Design review of the part built by this model. Coordinates are the model's own, in mm. Give positions to 0.01 mm unless a question says otherwise; leave off trailing zeros. Order: outer loops, then holes, each group sorted by start corner. A loop starts at its lowest first (then second) coordinate and runs counter-clockwise, first axis right, second up. Notation, with made-up numbers: M -26.5,82 L -18.5,82 A12 cw -18.5,86 Z; hole C 35.5,-8 d2. An arc over 180 degrees is marked long. Put each result on its own line as item: value. Start each with the question number.
Autodesk Inventor part; units mm, degrees
ref_plane "YZ Plane" through (0, 0, 0) normal (1, 0, 0) x (0, 1, 0)
ref_plane "XZ Plane" through (0, 0, 0) normal (0, 1, 0) x (-1, 0, 0)
ref_plane "XY Plane" through (0, 0, 0) normal (0, 0, 1) x (1, 0, 0)
sketch "Sketch1" plane through (0, 0, 0) normal (0, 0, 1) x (1, 0, 0)
  circle A0 centre (0, 0) radius 3.4
  line L0 (1.1333, -3.7357) -> (-1.1333, -3.7357)
  line L1 (-1.5333, -3.3357) -> (-1.5333, 3.3357)
  line L2 (-1.1333, 3.7357) -> (1.1333, 3.7357)
  line L3 (1.5333, 3.3357) -> (1.5333, -3.3357)
  line L4 (1.5333, -3.7357) -> (-1.5333, 3.7357) construction
  line L5 (-1.5333, -3.7357) -> (1.5333, 3.7357) construction
  arc A1 (-1.1333, 3.7357) -> (-1.5333, 3.3357) centre (-1.1333, 3.3357) ccw
  arc A2 (1.5333, 3.3357) -> (1.1333, 3.7357) centre (1.1333, 3.3357) ccw
  arc A3 (1.1333, -3.7357) -> (1.5333, -3.3357) centre (1.1333, -3.3357) ccw
  arc A4 (-1.5333, -3.3357) -> (-1.1333, -3.7357) centre (-1.1333, -3.3357) ccw
  point P0 (-1.5333, 3.0346)
  point P1 (-1.5333, -3.0346)
  point P2 (1.5333, -3.0346)
  point P3 (1.5333, 3.0346)
  point P4 (-0.9416, 2.2076)
  point P5 (-0.9416, -2.2076)
  point P6 (0.9416, -2.2076)
  point P7 (0.9416, 2.2076)
  dimension "d0" = 6.8
  dimension "d1" = 3.0667
  dimension "d2" = 7.4714
  dimension "d3" = 0.4
extrude "Extrusion1" add sketch "Sketch1" along normal blind 30
equation "\"d0\" = D_axel - d_toleransAxel"
equation "\"d3\" = r_filletAxel"
equation "\"d4\" = h_axel"
equation "\"D_axel\" = D_axel_1"
equation "\"d_axelRing\" = d_axelRing_1"
equation "\"r_filletAxel\" = r_filletAxel_1"
equation "\"d_toleransAxel\" = 0.2"
equation "\"h_axel\" = 30"
properties part number "Axel_parametriserad_03"
1. Consider section A-A on z = 25. Give the boundary of the cut face in (x, y).
2. Consider section B-B on y = 2.5. Give the boundary of the cut face in (x, z), then the cut area to 3 significant figures.
3. To check wall thickness, follow probe 1 along X at (y, z) = (0.25, 22.5); probe 2 along Y at (x, z) = (1.25, 4); probe 3 along Y at (x, z) = (2, 21.75). State the ranges of each line that lie inside material, in increasing order.
4. Consider section C-C on x = 2. Give the boundary of the cut face in (y, z).
Returned:
1. outline: M -1.53,-3.34 A0.4 ccw -1.13,-3.74 L 1.13,-3.74 A0.4 ccw 1.53,-3.34 L 1.53,-3.03 A3.4 ccw 1.53,3.03 L 1.53,3.34 A0.4 ccw 1.13,3.74 L -1.13,3.74 A0.4 ccw -1.53,3.34 L -1.53,3.03 A3.4 ccw -1.53,-3.03 Z
2. outline: M -2.3,0 L 2.3,0 L 2.3,30 L -2.3,30 Z
2. area: 138 mm2
3. probe 1: x = -3.39 to 3.39
3. probe 2: y = -3.72 to 3.72
3. probe 3: y = -2.75 to 2.75
4. outline: M -2.75,0 L 2.75,0 L 2.75,30 L -2.75,30 Z
